Check sheet for the modelled part. Datum: model origin and axes. Units: mm. Face numbers are marked on the shaded views. A direction names the side the tool comes from. Round coordinates to 2 decimals unless told otherwise and drop trailing zeros. Order: outer loops, then holes, each group sorted by start corner. A loop starts at its lowest first (then second) coordinate and runs counter-clockwise, first axis right, second up.
Q1. Cross-section at B-B on z = 4. Record the cut outline in (x, y) (3 decimals).
Q2. Scan lines: probe 1 along X at (y, z) = (1.2, 4.25); probe 2 along Y at (x, z) = (-3.75, 3); probe 3 along X at (y, z) = (-0.1, 5). Record each from-to range of solid material in increasing order.
Q3. Set-up check for the marked faces 5, 6 and 7: record each of +Z, -Z, +X, -X, +Y, -Y from which the full face is reachable in a straight line by a thin tool's end or side.
Q4. Cross-section at A-A on y = -0.8. Record the cut outline in (x, z) (3 decimals).
Q5. Depth check by flat-ended pin: P1, Ø2, axis at x = 1, y = 1.5, coming from the +Z side; P2, Ø4, axis at x = -7.175, z = 4, coming from the +Y side. Enter the tip coordinate at first touch or a pass-through.
Q6. Cross-section at C-C on y = 0.6. Give the number of separate pieces and of enclosed holes in the cut face, then the cut area to 3 significant figures.
Q7. Mould release check, pull along X, two halves, no side actions. Record for the marked faces 1, 2, 3 and 4: +X half, -X half, draft (parallel to the pull), parting line (faces both ways), or undercut.
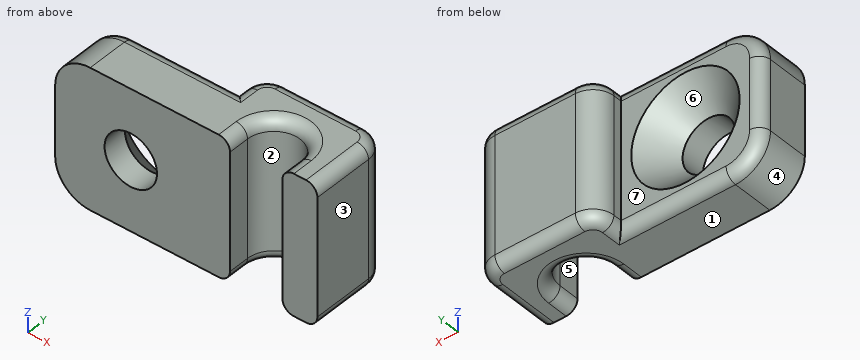
from build123d import *

# Parameters (mm, degrees)
RESSALTO_EXTRUS_O1_DEPTH = 8
ESBO_O2_R                = 1.5
CORTE_EXTRUS_O1_DEPTH    = 6
CHANFRO2_SIZE            = 1.6
FILETE3_R                = 2
FILETE5_R                = 1.2
FILETE6_R                = 0.65


with BuildPart() as part:
    # Esboço1 → Ressalto-extrusão1 (new body)
    with BuildSketch(Plane.XY):
        with BuildLine():
            Line((-11.5, -1.2), (-11.5, 1.8))
            Line((-11.5, 1.8), (-3.5, 1.8))
            Line((-3.5, 1.8), (-3.5, 3.5))
            Line((-3.5, 3.5), (3.5, 3.5))
            Line((3.5, 3.5), (3.5, -1.2))
            Line((3.5, -1.2), (1.5, -1.2))
            Line((1.5, -1.2), (1.5, 0))
            ThreePointArc((1.5, 0), (0, 1.5), (-1.5, 0))
            Line((-1.5, 0), (-1.5, -1.2))
            Line((-1.5, -1.2), (-11.5, -1.2))
        make_face()
    extrude(amount=RESSALTO_EXTRUS_O1_DEPTH)

    # Esboço2 → Corte-extrusão1 (cut)
    with BuildSketch(Plane(origin=(0, 1.8, 0), x_dir=(1, 0, 0), z_dir=(0, 1, 0))):
        with Locations(Location((-7.175, -4, 0), (0, 0, 180))):
            Circle(ESBO_O2_R)
    extrude(amount=-CORTE_EXTRUS_O1_DEPTH, mode=Mode.SUBTRACT)

    # Chanfro2
    chanfro2_edges = [part.edges().sort_by_distance(p)[0] for p in [
        (-5.675, 1.8, 4),
    ]]
    chamfer(chanfro2_edges, length=CHANFRO2_SIZE)

    # Filete3
    filete3_edges = [part.edges().sort_by_distance(p)[0] for p in [
        (-11.5, 0.3, 0),
        (-11.5, 0.3, 8),
    ]]
    fillet(filete3_edges, radius=FILETE3_R)

    # Filete5
    filete5_edges = [part.edges().sort_by_distance(p)[0] for p in [
        (-3.5, 3.5, 4),
        (3.5, 3.5, 4),
    ]]
    fillet(filete5_edges, radius=FILETE5_R)

    # Filete6
    filete6_edges = [part.edges().sort_by_distance(p)[0] for p in [
        (-1.5, -0.6, 0),
        (-6.5, 1.8, 0),
        (3.5, 0.55, 0),
        (1.5, -0.6, 0),
        (0, 1.5, 0),
        (3.5, 0.55, 8),
        (-6.5, 1.8, 8),
        (-1.5, -0.6, 8),
        (-11.5, 1.8, 4),
        (-10.914213562, 1.8, 0.585786438),
        (-10.914213562, 1.8, 7.414213562),
        (0, 1.5, 8),
        (-3.5, 2.05, 0),
        (-3.5, 2.05, 8),
        (0, 3.5, 0),
        (3.148528137, 3.148528137, 0),
        (-3.148528137, 3.148528137, 0),
        (0, 3.5, 8),
        (3.148528137, 3.148528137, 8),
        (-3.148528137, 3.148528137, 8),
        (1.5, -0.6, 8),
    ]]
    fillet(filete6_edges, radius=FILETE6_R)


solid = part.part
Results found:
1. outline: (-11.5, -1.2) - (-8.675, -1.2) - (-8.675, 0.2) - (-10.275, 1.8) - (-10.85, 1.8) arc R0.65 ccw to (-11.5, 1.15) - close; (-5.675, -1.2) - (-1.5, -1.2) - (-1.5, 0) arc R1.5 cw to (1.5, 0) - (1.5, -1.2) - (3.5, -1.2) - (3.5, 2.3) arc R1.2 ccw to (2.3, 3.5) - (-2.3, 3.5) arc R1.2 ccw to (-3.5, 2.3) - (-3.5, 1.8) - (-4.075, 1.8) - (-5.675, 0.2) - close
2. probe 1: x = -11.5 to -9.66, -4.69 to -0.9, 0.9 to 3.5
2. probe 2: y = -1.2 to 1.8
2. probe 3: x = -11.5 to -8.29, -6.06 to -1.5, 1.5 to 3.5
3. face 5: +Z, -Z, -Y
3. face 6: +Y
3. face 7: +Z, -Z, -X, +Y
4. outline: (-11.5, 2) arc R2 ccw to (-9.5, 0) - (-2.15, 0) arc R0.65 ccw to (-1.5, 0.65) - (-1.5, 7.35) arc R0.65 ccw to (-2.15, 8) - (-9.5, 8) arc R2 ccw to (-11.5, 6) - close; (1.5, 0.65) arc R0.65 ccw to (2.15, 0) - (2.85, 0) arc R0.65 ccw to (3.5, 0.65) - (3.5, 7.35) arc R0.65 ccw to (2.85, 8) - (2.15, 8) arc R0.65 ccw to (1.5, 7.35) - close; hole circle Ø3 at (-7.175, 4)
5. P1: stops at z = 8
5. P2: stops at y = 0.7
6. separate pieces: 2
6. enclosed holes: 1
6. area: 84.4 mm2
7. face 1: draft
7. face 2: undercut
7. face 3: +X half
7. face 4: -X half
